The listing builds one solid part. Answer for the finished solid, in the listing's coordinates (mm). A direction names the side the tool comes from. Coordinates: 2 decimals unless noted, no trailing zeros. Order: outer loops, then holes, each group sorted by start corner. A loop starts at its lowest first (then second) coordinate and runs counter-clockwise, first axis right, second up. Notation, with made-up numbers: (-30, 44) - (-17, 44) arc R25 cw to (-17, 82) - close; hole circle Ø10 at (63.25, 23.25). An arc over 180 degrees is marked (long way). Use a Markdown table: item, result. Add a question column.
Item 1: For faces 1 (the flat face through (0, 0, -0.45)), 2 (the flat face through (8.26, -0.01, 2.99)), determine the directions among +Z, -Z, +X, -X, +Y, -Y from which every point of the face is accessible in a straight line to the end or side of a thin tool.
Item 2: Find the intervals of material crossed by line 1 along Z through (x, y) = (3, -0.3); line 2 along X through (y, z) = (0.6, -1.75), in increasing order.
Item 3: The part is cut by section C-C, the plane x = -3.75. Give the vertices of the cut face in (y, z) (3 decimals).
Item 4: The part is cut by section B-B, the plane y = 0.5. Give the vertices of the cut face in (x, z).
Item 5: The part is cut by section D-D, the plane x = -6.5. Give the vertices of the cut face in (y, z) (3 decimals).
Item 6: The part is cut by section A-A, the plane z = -1.5. Give the vertices of the cut face in (x, y) (3 decimals).
from build123d import *

# Parameters (mm, degrees)
SKIZZE1_W                       = 18
SKIZZE1_H                       = 7.5
SKIZZE1_W_2                     = 14
SKIZZE1_H_2                     = 1.7
AUFSATZ_LINEAR_AUSTRAGEN1_DEPTH = 0.825
VERRUNDUNG1_R                   = 0.8
FASE1_SIZE                      = 1.5


with BuildPart() as part:
    # Skizze1 → Aufsatz-Linear austragen1 (new body, symmetric)
    with BuildSketch(Plane(origin=(0, 0, 0), x_dir=(1, 0, 0), z_dir=(0, 1, 0))):
        Rectangle(SKIZZE1_W, SKIZZE1_H)
        with Locations((0, -1.3)):
            Rectangle(SKIZZE1_W_2, SKIZZE1_H_2, mode=Mode.SUBTRACT)
        with BuildLine():
            Line((-6, 2.55), (6, 2.55))
            ThreePointArc((6, 2.55), (7.05, 1.5), (6, 0.45))
            Line((6, 0.45), (-6, 0.45))
            ThreePointArc((-6, 0.45), (-7.05, 1.5), (-6, 2.55))
        make_face(mode=Mode.SUBTRACT)
    extrude(amount=AUFSATZ_LINEAR_AUSTRAGEN1_DEPTH, both=True)

    # Verrundung1
    verrundung1_edges = [part.edges().sort_by_distance(p)[0] for p in [
        (-7, 0, 2.15),
        (-7, 0, 0.45),
        (7, 0, 0.45),
        (7, 0, 2.15),
    ]]
    fillet(verrundung1_edges, radius=VERRUNDUNG1_R)

    # Fase1
    fase1_edges = [part.edges().sort_by_distance(p)[0] for p in [
        (9, 0, 3.75),
        (-9, 0, 3.75),
    ]]
    chamfer(fase1_edges, length=FASE1_SIZE)


solid = part.part
Solution:
| question | item | result |
|---|---|---|
| 1 | face 1 | +Y, -Y |
| 1 | face 2 | +Z, +X, +Y, -Y |
| 2 | line 1 | z = -3.75 to -2.55, -0.45 to 0.45, 2.15 to 3.75 |
| 2 | line 2 | x = -9 to -7.02, 7.02 to 9 |
| 3 | outline | (-0.825, -3.75) - (0.825, -3.75) - (0.825, -2.55) - (-0.825, -2.55) - close; (-0.825, -0.45) - (0.825, -0.45) - (0.825, 0.45) - (-0.825, 0.45) - close; (-0.825, 2.15) - (0.825, 2.15) - (0.825, 3.75) - (-0.825, 3.75) - close |
| 4 | outline | (-9, -3.75) - (9, -3.75) - (9, 2.25) - (7.5, 3.75) - (-7.5, 3.75) - (-9, 2.25) - close; hole (-7, 1.25) arc R0.8 ccw to (-6.2, 0.45) - (6.2, 0.45) arc R0.8 ccw to (7, 1.25) - (7, 1.35) arc R0.8 ccw to (6.2, 2.15) - (-6.2, 2.15) arc R0.8 ccw to (-7, 1.35) - close; hole (-6, -2.55) - (6, -2.55) arc R1.05 ccw to (6, -0.45) - (-6, -0.45) arc R1.05 ccw to start |
| 5 | outline | (-0.825, -3.75) - (0.825, -3.75) - (0.825, -2.423) - (-0.825, -2.423) - close; (-0.825, -0.577) - (0.825, -0.577) - (0.825, 0.508) - (-0.825, 0.508) - close; (-0.825, 2.092) - (0.825, 2.092) - (0.825, 3.75) - (-0.825, 3.75) - close |
| 6 | outline | (-9, -0.825) - (-7.05, -0.825) - (-7.05, 0.825) - (-9, 0.825) - close; (7.05, -0.825) - (9, -0.825) - (9, 0.825) - (7.05, 0.825) - close |
